Here's how the part is built. I have some questions about the finished solid (model axes, mm). A direction names the side the tool comes from. Coordinates: 2 decimals unless noted, no trailing zeros. Loops run counter-clockwise (first coordinate to the right, second up) from the corner with the lowest first, then second, coordinate; pieces in that order, holes last. Notation, with made-up numbers: (37.5, 28) -> (70.5, 28) arc R16 ccw to (70.5, 32) -> close; hole circle Ø7 at (-32, 87.5). An arc over 180 degrees is marked (long way). Answer as a JSON object with one key per item and string values. Group by question number.
Q1. On a 3-axis mill with a long thin cutter (end or side, diameter ignored), from which of +Z, -Z, +X, -X, +Y, -Y can I reach the whole of each face in a straight line? I mean faces 5 (the flat face through (6, 22.5, 10)), 6 (the flat face through (6, -2, 10)), 7 (the flat face through (-2, 5, 10)). Say none if no direction works.
Q2. I want a section at B-B on x = 4. Write out the boundary of the cut face in (y, z).
Q3. Thinking about a two-plate mould opening in X: for faces 1 (the flat face through (7, 11, 20)), 2 (the flat face through (14.5, 5, 10)), 3 (the flat face through (6, 13.5, 10)), 4 (the flat face through (-6.023, 17.937, 9.86)), which applies, released by +X, released by -X, zero draft, split by the parting line, or undercut?
Q4. I need wall thicknesses on line 1 (Y direction, x = 5, z = 17.5); line 2 (X direction, y = 1.75, z = 2.75); line 3 (X direction, y = 11, z = 3.5). Which ranges of each line are inside material? Lowest first, please.
Q5. I want a section at C-C on x = 13. Write out the boundary of the cut face in (y, z).
Q6. I want a section at D-D on z = 2.75. Write out the boundary of the cut face in (x, y).
Q7. I want a section at A-A on y = 9.25. Write out the boundary of the cut face in (x, z).
Q8. I'm going to push flat-ended pins straight in: pin 1 (11.5 mm diameter, centred on y = 5, z = 12, fed in from -X); pin 2 (11.5 mm diameter, centred on y = 2.5, z = 9.5, fed in from +X); pin 3 (5 mm diameter, centred on x = 18.5, z = 6, fed in from -Y). Where does each tip first touch, or does it pass through?
```python
from build123d import *

# Parameters (mm, degrees)
SKETCH1_W           = 16.5
SKETCH1_H           = 14.5
SKETCH1_W_2         = 12.5
SKETCH1_H_2         = 10.5
BOSS_EXTRUDE1_DEPTH = 20
BOSS_EXTRUDE2_DEPTH = 20


with BuildPart() as part:
    # Sketch1 → Boss-Extrude1 (new body)
    with BuildSketch(Plane.XY):
        with Locations((6.25, 5.25)):
            Rectangle(SKETCH1_W, SKETCH1_H)
        with Locations((6.25, 5.25)):
            Rectangle(SKETCH1_W_2, SKETCH1_H_2, mode=Mode.SUBTRACT)
    extrude(amount=BOSS_EXTRUDE1_DEPTH)

    # Sketch2 → Boss-Extrude2 (add)
    with BuildSketch(Plane(origin=(0, 0, 0), x_dir=(-1, 0, 0), z_dir=(0, 0, -1))):
        Polygon((2, 12.5), (13, 23.5), (-24.907922473, 23.5), (-14.5, 12.5), align=None)
        Polygon((-22.585068112, 22.5), (-14.069495179, 13.5), (1.585786438, 13.5), (10.585786438, 22.5), align=None, mode=Mode.SUBTRACT)
    extrude(amount=-BOSS_EXTRUDE2_DEPTH)


solid = part.part
```
Result set:
{
 "1": {"face 5": "+Z, -Z", "face 6": "+Z, -Z, +X, -X, -Y", "face 7": "+Z, -Z, -X, -Y"},
 "2": {"outline": "(-2, 0) -> (0, 0) -> (0, 20) -> (-2, 20) -> close; (10.5, 0) -> (13.5, 0) -> (13.5, 20) -> (10.5, 20) -> close; (22.5, 0) -> (23.5, 0) -> (23.5, 20) -> (22.5, 20) -> close"},
 "3": {"face 1": "zero draft", "face 2": "released by +X", "face 3": "undercut", "face 4": "undercut"},
 "4": {"line 1": "y = -2 to 0, 10.5 to 13.5, 22.5 to 23.5", "line 2": "x = -2 to 0, 12.5 to 14.5", "line 3": "x = -2 to 14.5"},
 "5": {"outline": "(-2, 0) -> (13.5, 0) -> (13.5, 20) -> (-2, 20) -> close; (22.5, 0) -> (23.5, 0) -> (23.5, 20) -> (22.5, 20) -> close"},
 "6": {"outline": "(-13, 23.5) -> (-2, 12.5) -> (-2, -2) -> (14.5, -2) -> (14.5, 12.5) -> (24.91, 23.5) -> close; hole (-10.59, 22.5) -> (-1.59, 13.5) -> (14.07, 13.5) -> (22.59, 22.5) -> close; hole (0, 0) -> (12.5, 0) -> (12.5, 10.5) -> (0, 10.5) -> close"},
 "7": {"outline": "(-2, 0) -> (0, 0) -> (0, 20) -> (-2, 20) -> close; (12.5, 0) -> (14.5, 0) -> (14.5, 20) -> (12.5, 20) -> close"},
 "8": {"pin 1": "stops at x = -2", "pin 2": "stops at x = 14.5", "pin 3": "stops at y = 14.09"}
}
